Source: CAD feature listing. Evaluate the final solid. Frame: model axes, mm. Face numbers are marked on the shaded views. Give positions to 0.01 mm unless a question says otherwise; leave off trailing zeros. Loops run counter-clockwise (first coordinate to the right, second up) from the corner with the lowest first, then second, coordinate; pieces in that order, holes last. Notation, with made-up numbers: M 66,19 L 76,19 A36 ccw 76,58 Z; hole C 88.25,85.5 d9. An arc over 180 degrees is marked long. Answer in a Markdown table with one row per item.
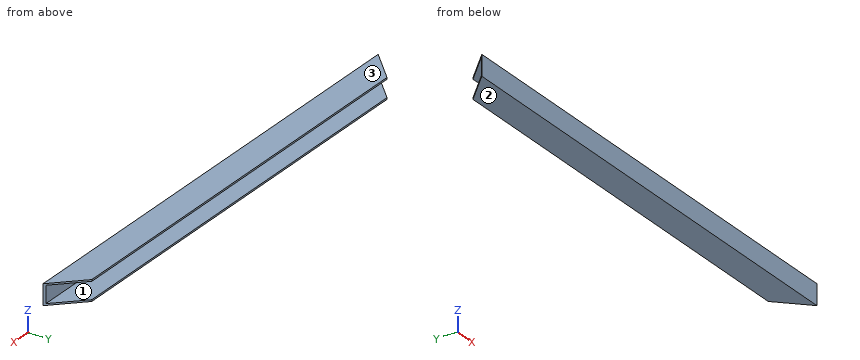
```python
from build123d import *

# Parameters (mm, degrees)
F0_W       = 69
F0_H       = 49
F1_DEPTH   = 579
F2_T       = -4
F3_C1_SIZE = 68.9999
F3_C2_SIZE = 68.9999


# Not quite as in the source:
# - a fillet or chamfer is up to 0.001 mm smaller than in the source, because OpenCascade refuses the exact size


with BuildPart() as f1:
    # F0 (on Right) → F1 (new body, symmetric)
    with BuildSketch(Plane.YZ):
        Rectangle(F0_W, F0_H)
    extrude(amount=F1_DEPTH, both=True)

    # F2
    f2_openings = [f1.faces().sort_by_distance(p)[0] for p in [
        (579, 0, 0),
        (0, 34.5, 0),
        (-579, 0, 0),
    ]]
    offset(amount=F2_T, openings=f2_openings)

    # F3: chamfer of 69 on 4 edges, made by hand

    # F3_c1 (size 69 in the source; OpenCascade refuses exactly that, so slightly less here)
    f3_c1_edges = [f1.edges().sort_by_distance(p)[0] for p in [
        (579, 34.5, -22.5),
    ]]
    chamfer(f3_c1_edges, length=F3_C1_SIZE)

    # F3_c2 (size 69 in the source; OpenCascade refuses exactly that, so slightly less here)
    f3_c2_edges = [f1.edges().sort_by_distance(p)[0] for p in [
        (-579, 34.5, -22.5),
    ]]
    chamfer(f3_c2_edges, length=F3_C2_SIZE)


solid = f1.part
```
1) Pull-direction query (Z, two-part tool) for the marked faces 1, 2 and 3; classes: released by +Z, released by -Z, zero draft, split by the parting line, or undercut.
Reply:
| item | result |
|---|---|
| face 1 | undercut |
| face 2 | released by -Z |
| face 3 | released by +Z |
2) Material intervals for L1, parallel to Z at x = 216.5, y = -2.5; L2, parallel to Y at x = -410, z = -15.5, sorted ascending.
Reply:
| item | result |
|---|---|
| L1 | z = -24.5 to -20.5, 20.5 to 24.5 |
| L2 | y = -34.5 to -30.5 |
3) Pin query (flat end, axial travel): pin 1 Ø8 at (x, z) = (33.5, 17) entering from +Y; pin 2 Ø20.5 at (x, z) = (-256.5, -1.5) entering from +Y. Return the tip coordinate at first contact, or that it passes through.
Reply:
| item | result |
|---|---|
| pin 1 | stops at y = 34.5 |
| pin 2 | stops at y = -30.5 |
4) Section D-D, the plane y = -18. Return loops of the section in (x, z).
Reply:
| item | result |
|---|---|
| outline | M -562.5,-24.5 L 562.5,-24.5 L 562.5,-20.5 L -562.5,-20.5 Z; M -562.5,20.5 L 562.5,20.5 L 562.5,24.5 L -562.5,24.5 Z |
5) Section B-B, the plane x = 257. Return loops of the section in (y, z), then the cut area to 3 significant figures.
Reply:
| item | result |
|---|---|
| outline | M -34.5,-24.5 L 34.5,-24.5 L 34.5,-20.5 L -30.5,-20.5 L -30.5,20.5 L 34.5,20.5 L 34.5,24.5 L -34.5,24.5 Z |
| area | 716 mm² |
6) Section A-A, the plane y = 23.5. Return loops of the section in (x, z).
Reply:
| item | result |
|---|---|
| outline | M -521,-24.5 L 521,-24.5 L 521,-20.5 L -521,-20.5 Z; M -521,20.5 L 521,20.5 L 521,24.5 L -521,24.5 Z |
